```python
from build123d import *

# Parameters (mm, degrees)
F0_W     = 25.4
F0_H     = 50.8
F1_DEPTH = 50.8
F2_R     = 12.7


with BuildPart() as f1:
    # F0 (on Front) → F1 (new body)
    with BuildSketch(Plane.XZ):
        Polygon((527.929086, 304.8), (0, 0), (0, -50.8), (527.929086, 254), align=None)
        with Locations((540.629086, 279.4)):
            Rectangle(F0_W, F0_H)
    extrude(amount=F1_DEPTH)

    # F2
    f2_edges = [f1.edges().sort_by_distance(p)[0] for p in [
        (263.964543, -50.8, 152.4),
        (263.964543, -50.8, 101.6),
        (263.964543, 0, 152.4),
        (263.964543, 0, 101.6),
    ]]
    fillet(f2_edges, radius=F2_R)


solid = f1.part
```
Geometry check sheet. Reference: the model listing, model coordinates, mm. Give positions to 0.01 mm unless a question says otherwise; leave off trailing zeros. Write each loop counter-clockwise with the first axis right and the second up, starting at its lowest first coordinate (ties: lowest second). Pieces come first, ordered by that corner, then holes.
1) Material ranges on L1, parallel to Z at x = 472, y = -41.5; L2, parallel to X at y = -45, z = 273; L3, parallel to Z at x = 238, y = -20.5, recorded low to high.
2) Gauge pin test, flat ends, axial feed: pin 1 (10 mm diameter, centred on x = 79, y = -30, fed in from -Z); pin 2 (12 mm diameter, centred on x = 233.5, y = -31.5, fed in from +Z); pin 3 (2 mm diameter, centred on y = -27.5, z = 193, fed in from -X). Record the tip position at first contact, or that the pin passes through.
3) Section check A-A, the plane y = -26.5. Record the boundary of the cut face in (x, z).
Computed:
1. L1: z = 222.24 to 271.97
1. L2: x = 476.93 to 553.33
1. L3: z = 86.61 to 137.41
2. pin 1: stops at z = -8.08
2. pin 2: stops at z = 138.28
2. pin 3: stops at x = 332.55
3. outline: (0, -50.8) - (527.93, 254) - (553.33, 254) - (553.33, 304.8) - (527.93, 304.8) - (0, 0) - close
